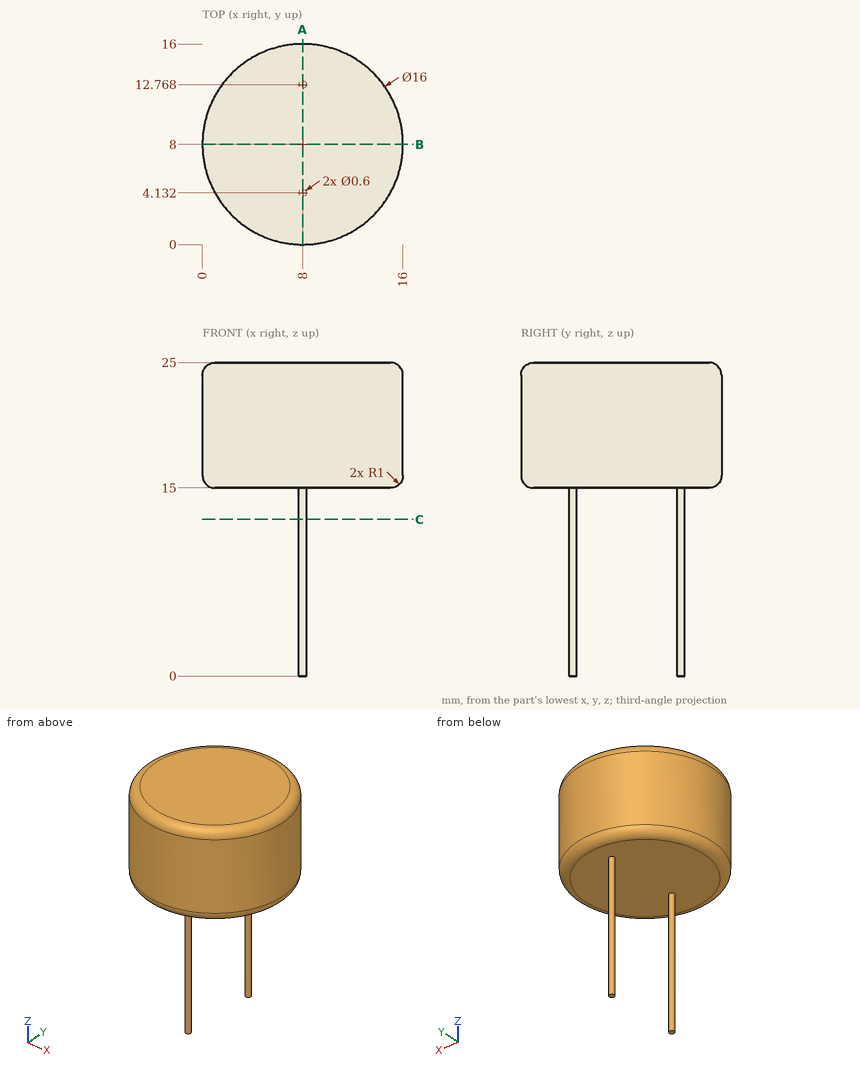
Drawing for the job (mm, zero at the part's lowest x, y, z). Give positions to 0.01 mm unless a question says otherwise; leave off trailing zeros. Order: outer loops, then holes, each group sorted by start corner. A loop starts at its lowest first (then second) coordinate and runs counter-clockwise, first axis right, second up. Notation, with made-up numbers: (67, 38.25) - (105, 38.25) arc R23 ccw to (105, 68.25) - close; hole circle Ø7 at (27, -16). An arc over 180 degrees is marked (long way). Use one line per item in the form item = value.
Item 1: Probe probe 1 along Z at (x, y) = (9, 10.75); probe 2 along Z at (x, y) = (12.75, 2.25); probe 3 along Y at (x, z) = (4.5, 15.25) (1 decimal). List the from-to ranges inside material, lowest first. Write a range as from..to.
Solution:
probe_1 = 15..25
probe_2 = 15.11..24.89
probe_3 = 1.2..14.8
Item 2: Pin check, flat tips, straight feed: pin 1 Ø5 at (y, z) = (6, 17) entering from -X; pin 2 Ø6 at (x, y) = (13, 13.5) entering from -Z; pin 3 Ø8 at (y, z) = (3, 20.5) entering from +X; pin 4 Ø1.5 at (x, z) = (5, 21.5) entering from +Y. Stop position of each tip, or through.
Solution:
pin_1 = 0
pin_2 = 15
pin_3 = 15.94
pin_4 = 15.68
Item 3: Slice it at C-C on z = 12.5. Give the cut face in (x, y).
Solution:
outline = circle Ø0.6 at (8, 4.13); circle Ø0.6 at (8, 12.77)
Item 4: Slice it at A-A on x = 8. Give the cut face in (y, z).
Solution:
outline = (0, 16) arc R1 ccw to (1, 15) - (3.83, 15) - (3.83, 0) - (4.43, 0) - (4.43, 15) - (12.47, 15) - (12.47, 0) - (13.07, 0) - (13.07, 15) - (15, 15) arc R1 ccw to (16, 16) - (16, 24) arc R1 ccw to (15, 25) - (1, 25) arc R1 ccw to (0, 24) - close
Item 5: Slice it at B-B on y = 8. Give the cut face in (x, z), and give its area (3 significant figures).
Solution:
outline = (0, 16) arc R1 ccw to (1, 15) - (15, 15) arc R1 ccw to (16, 16) - (16, 24) arc R1 ccw to (15, 25) - (1, 25) arc R1 ccw to (0, 24) - close
area = 159 mm2
